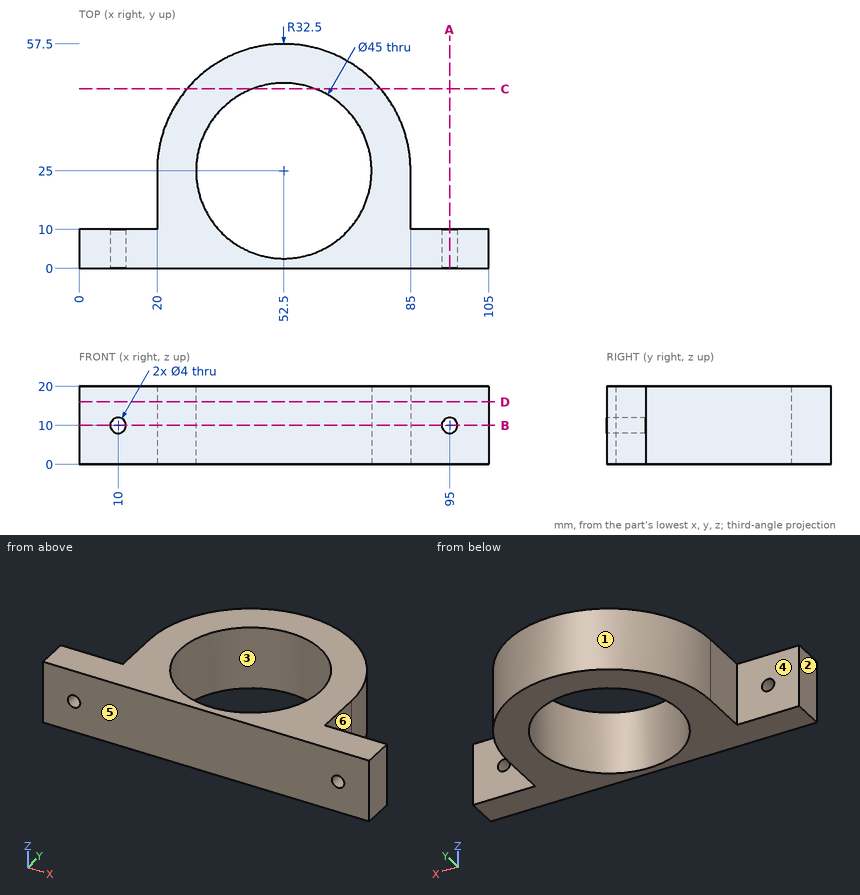
Source: three-view drawing plus pictorial views. Frame: mm from the lowest corner of the part. A direction names the side the tool comes from. Give positions to 0.01 mm unless a question says otherwise; leave off trailing zeros. Order: outer loops, then holes, each group sorted by start corner. A loop starts at its lowest first (then second) coordinate and runs counter-clockwise, first axis right, second up. Notation, with made-up numbers: (12, 63) -> (20, 63) arc R7 ccw to (20, 70) -> close; hole circle Ø2 at (13, 31.25). An arc over 180 degrees is marked (long way). Use a Markdown table: item, result.
Q1. Section C-C (y = 46). Return the cut outline in (x, z), and give its area (3 significant figures).
A:
| item | result |
|---|---|
| outline | (27.7, 0) -> (44.42, 0) -> (44.42, 20) -> (27.7, 20) -> close; (60.58, 0) -> (77.3, 0) -> (77.3, 20) -> (60.58, 20) -> close |
| area | 669 mm^2 |
Q2. Access query for the marked faces 4, 5 and 6. Directions: +Z, -Z, +X, -X, +Y, -Y. A direction counts if a zero-diameter tool reaches every point of the face in a straight line with its end or side. Return the directions, or none.
A:
| item | result |
|---|---|
| face 4 | +Z, -Z, -X, +Y |
| face 5 | +Z, -Z, +X, -X, -Y |
| face 6 | +Z, -Z, +X, +Y |
Q3. Section B-B (z = 10). Return the cut outline in (x, y).
A:
| item | result |
|---|---|
| outline | (0, 0) -> (8, 0) -> (8, 10) -> (0, 10) -> close; (12, 0) -> (93, 0) -> (93, 10) -> (85, 10) -> (85, 25) arc R32.5 ccw to (20, 25) -> (20, 10) -> (12, 10) -> close; (97, 0) -> (105, 0) -> (105, 10) -> (97, 10) -> close; hole circle Ø45 at (52.5, 25) |
Q4. Material intervals for line 1 (Z direction, x = 95, y = 4); line 2 (Y direction, x = 52.5, z = 13.75); line 3 (X direction, y = 5.25, z = 10), sorted ascending. Write a range as [from, to].
A:
| item | result |
|---|---|
| line 1 | [0, 8], [12, 20] |
| line 2 | [0, 2.5], [47.5, 57.5] |
| line 3 | [0, 8], [12, 41.72], [63.28, 93], [97, 105] |
Q5. Section A-A (x = 95). Return the cut outline in (y, z), and give its area (3 significant figures).
A:
| item | result |
|---|---|
| outline | (0, 0) -> (10, 0) -> (10, 8) -> (0, 8) -> close; (0, 12) -> (10, 12) -> (10, 20) -> (0, 20) -> close |
| area | 160 mm^2 |
Q6. First-contact query: P1, Ø8, axis at y = 49.5, z = 13.5, coming from the +X side; P2, Ø12, axis at y = 21, z = 15, coming from the -X side; P3, Ø7.5, axis at y = 19, z = 7, coming from the +X side. Flat tips, straight axial feed; report the tip coordinate or a pass-through.
A:
| item | result |
|---|---|
| P1 | x = 77.72 |
| P2 | x = 20 |
| P3 | x = 85 |
Q7. Pull-direction query (X, two-part tool) for the marked faces 1, 2 and 3; classes: +X half, -X half, draft (parallel to the pull), parting line (faces both ways), or undercut.
A:
| item | result |
|---|---|
| face 1 | parting line |
| face 2 | -X half |
| face 3 | undercut |
Q8. Section D-D (z = 16). Return the cut outline in (x, y), and give its area (3 significant figures).
A:
| item | result |
|---|---|
| outline | (0, 0) -> (105, 0) -> (105, 10) -> (85, 10) -> (85, 25) arc R32.5 ccw to (20, 25) -> (20, 10) -> (0, 10) -> close; hole circle Ø45 at (52.5, 25) |
| area | 2,090 mm^2 |
